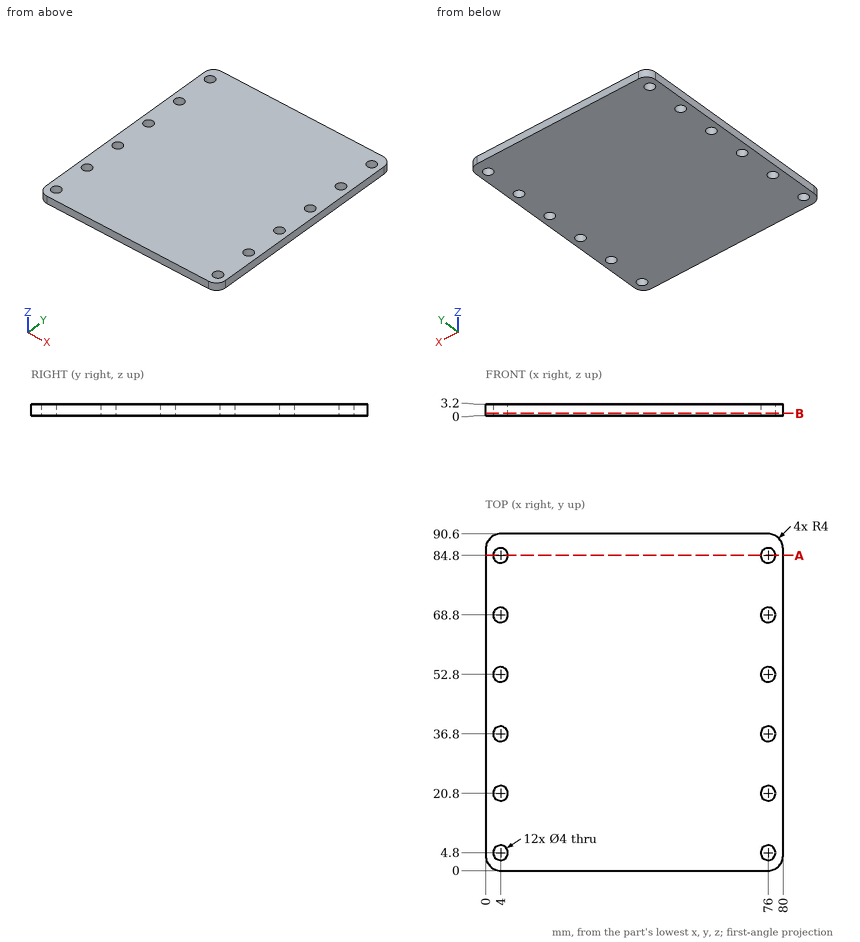
Design review of the part shown in the three views and the two pictorial views. Dimensions are in mm from the part's minimum x, y and z. Give positions to 0.01 mm unless a question says otherwise; leave off trailing zeros. Loops run counter-clockwise (first coordinate to the right, second up) from the corner with the lowest first, then second, coordinate; pieces in that order, holes last. Notation, with made-up numbers: (79, 13.5) -> (136, 13.5) arc R24 cw to (136, 24.5) -> close; hole circle Ø8 at (51, 21.5). An arc over 180 degrees is marked (long way). Write each question's results on one line, items separated by ' | '.
Q1. For pin 1 Ø3.5 at (x, y) = (4, 36.8) entering from +Z, flat-tipped, find the tip position at first contact; note if it passes through.
Reply:
pin 1: passes through
Q2. Take a section at A-A, the plane y = 84.8. Write out the cut boundary in (x, z).
Reply:
outline: (0, 0) -> (2, 0) -> (2, 3.2) -> (0, 3.2) -> close; (6, 0) -> (74, 0) -> (74, 3.2) -> (6, 3.2) -> close; (78, 0) -> (80, 0) -> (80, 3.2) -> (78, 3.2) -> close
Q3. Take a section at B-B, the plane z = 0.7. Give the number of separate pieces and of enclosed holes in the cut face, plus the area to 3 significant figures.
Reply:
separate pieces: 1 | enclosed holes: 12 | area: 7,080 mm²
Q4. Wall thickness on L1, parallel to X at y = 35, z = 2.2: over which ranges is the line inside the solid? List them lowest first.
Reply:
L1: x = 0 to 3.13, 4.87 to 75.13, 76.87 to 80
